from build123d import *

# Parameters (mm, degrees)
SKETCH_1_W      = 20
SKETCH_1_H      = 25
EXTRUDE_1_DEPTH = 4
FILLET_2_R      = 1
FILLET_3_R      = 1


with BuildPart() as part:
    # 草图1 → 凸台-拉伸1 (new body)
    with BuildSketch(Plane(origin=(0, 0, 0), x_dir=(1, 0, 0), z_dir=(0, 1, 0))):
        Rectangle(SKETCH_1_W, SKETCH_1_H)
    extrude(amount=EXTRUDE_1_DEPTH)

    # 圆角2
    fillet_2_edges = [part.edges().sort_by_distance(p)[0] for p in [
        (-10, 4, 0),
        (0, 0, 12.5),
        (-10, 0, 0),
        (0, 0, -12.5),
        (10, 0, 0),
        (-10, 2, 12.5),
        (-10, 2, -12.5),
    ]]
    fillet(fillet_2_edges, radius=FILLET_2_R)

    # 圆角3
    # the kernel refuses this fillet: 1 mm, written as the material it takes off along each edge
    with BuildSketch(Plane(origin=(-9, 3, 11.5), x_dir=(0, 0, 1), z_dir=(0, 1, 0))) as fillet_3_piece_1_section:
        Polygon((0, 0), (FILLET_3_R, 0), (FILLET_3_R, -FILLET_3_R), (0, -FILLET_3_R), align=None)
    fillet_3_piece_1 = extrude(amount=FILLET_3_R, mode=Mode.PRIVATE)
    fillet_3_piece_1 = fillet_3_piece_1 - Plane(origin=(-9, 3, 11.5), x_dir=(0.7071067811865475, 0, -0.7071067811865477), z_dir=(0, 1, 0)) * Sphere(FILLET_3_R, mode=Mode.PRIVATE)
    add(fillet_3_piece_1, mode=Mode.SUBTRACT)
    with BuildSketch(Plane(origin=(-9, 3, -11.5), x_dir=(0, 1, 0), z_dir=(0, 0, -1))) as fillet_3_piece_2_section:
        Polygon((0, 0), (FILLET_3_R, 0), (FILLET_3_R, -FILLET_3_R), (0, -FILLET_3_R), align=None)
    fillet_3_piece_2 = extrude(amount=FILLET_3_R, mode=Mode.PRIVATE)
    fillet_3_piece_2 = fillet_3_piece_2 - Plane(origin=(-9, 3, -11.5), x_dir=(0.7071067811865475, -0.7071067811865475, 0), z_dir=(0, 0, -1)) * Sphere(FILLET_3_R, mode=Mode.PRIVATE)
    add(fillet_3_piece_2, mode=Mode.SUBTRACT)
    with BuildSketch(Plane(origin=(9, 1, 11.5), x_dir=(0, 0, 1), z_dir=(1, 0, 0))) as fillet_3_piece_3_section:
        Polygon((0, 0), (FILLET_3_R, 0), (FILLET_3_R, FILLET_3_R), (0, FILLET_3_R), align=None)
    fillet_3_piece_3 = extrude(amount=FILLET_3_R, mode=Mode.PRIVATE)
    fillet_3_piece_3 = fillet_3_piece_3 - Plane(origin=(9, 1, 11.5), x_dir=(0, 0.7071067811865475, -0.7071067811865475), z_dir=(1, 0, 0)) * Sphere(FILLET_3_R, mode=Mode.PRIVATE)
    add(fillet_3_piece_3, mode=Mode.SUBTRACT)
    with BuildSketch(Plane(origin=(9, 1, -11.5), x_dir=(1, 0, 0), z_dir=(0, 0, -1))) as fillet_3_piece_4_section:
        Polygon((0, 0), (FILLET_3_R, 0), (FILLET_3_R, FILLET_3_R), (0, FILLET_3_R), align=None)
    fillet_3_piece_4 = extrude(amount=FILLET_3_R, mode=Mode.PRIVATE)
    fillet_3_piece_4 = fillet_3_piece_4 - Plane(origin=(9, 1, -11.5), x_dir=(-0.7071067811865475, 0.7071067811865475, 0), z_dir=(0, 0, -1)) * Sphere(FILLET_3_R, mode=Mode.PRIVATE)
    add(fillet_3_piece_4, mode=Mode.SUBTRACT)
    with BuildSketch(Plane(origin=(9, 3, 11.5), x_dir=(0, 1, 0), z_dir=(1, 0, 0))) as fillet_3_piece_5_section:
        Polygon((0, 0), (FILLET_3_R, 0), (FILLET_3_R, FILLET_3_R), (0, FILLET_3_R), align=None)
    fillet_3_piece_5 = extrude(amount=FILLET_3_R, mode=Mode.PRIVATE)
    fillet_3_piece_5 = fillet_3_piece_5 - Plane(origin=(9, 3, 11.5), x_dir=(0, -0.7071067811865475, -0.7071067811865475), z_dir=(1, 0, 0)) * Sphere(FILLET_3_R, mode=Mode.PRIVATE)
    add(fillet_3_piece_5, mode=Mode.SUBTRACT)
    with BuildSketch(Plane(origin=(9, 3, -11.5), x_dir=(1, 0, 0), z_dir=(0, 0, -1))) as fillet_3_piece_6_section:
        Polygon((0, 0), (FILLET_3_R, 0), (FILLET_3_R, -FILLET_3_R), (0, -FILLET_3_R), align=None)
    fillet_3_piece_6 = extrude(amount=FILLET_3_R, mode=Mode.PRIVATE)
    fillet_3_piece_6 = fillet_3_piece_6 - Plane(origin=(9, 3, -11.5), x_dir=(-0.7071067811865475, -0.7071067811865475, 0), z_dir=(0, 0, -1)) * Sphere(FILLET_3_R, mode=Mode.PRIVATE)
    add(fillet_3_piece_6, mode=Mode.SUBTRACT)
    with BuildSketch(Plane(origin=(9, 4, 12.5), x_dir=(0, 0, -1), z_dir=(-1, 0, 0))) as fillet_3_piece_7:
        with BuildLine():
            CenterArc((FILLET_3_R, FILLET_3_R), FILLET_3_R, 180, 90)
            Line((0, FILLET_3_R), (0, 0))
            Line((0, 0), (FILLET_3_R, 0))
        make_face()
    extrude(amount=18, mode=Mode.SUBTRACT)
    with BuildSketch(Plane(origin=(10, 4, -11.5), x_dir=(0, -1, 0), z_dir=(0, 0, 1))) as fillet_3_piece_8:
        with BuildLine():
            CenterArc((FILLET_3_R, -FILLET_3_R), FILLET_3_R, 90, 90)
            Line((0, -FILLET_3_R), (0, 0))
            Line((0, 0), (FILLET_3_R, 0))
        make_face()
    extrude(amount=23, mode=Mode.SUBTRACT)
    with BuildSketch(Plane(origin=(-9, 4, -12.5), x_dir=(0, -1, 0), z_dir=(1, 0, 0))) as fillet_3_piece_9:
        with BuildLine():
            CenterArc((FILLET_3_R, -FILLET_3_R), FILLET_3_R, 90, 90)
            Line((0, -FILLET_3_R), (0, 0))
            Line((0, 0), (FILLET_3_R, 0))
        make_face()
    extrude(amount=18, mode=Mode.SUBTRACT)
    with BuildSketch(Plane(origin=(10, 1, 12.5), x_dir=(0, 0, -1), z_dir=(0, 1, 0)), Plane(origin=(10, 1, -12.5), x_dir=(-1, 0, 0), z_dir=(0, 1, 0))) as fillet_3_piece_10:
        with BuildLine():
            CenterArc((FILLET_3_R, FILLET_3_R), FILLET_3_R, 180, 90)
            Line((0, FILLET_3_R), (0, 0))
            Line((0, 0), (FILLET_3_R, 0))
        make_face()
    extrude(amount=2, mode=Mode.SUBTRACT)


solid = part.part
Here's how the part is built. I have some questions about the finished solid (model axes, mm). Coordinates: 2 decimals unless noted, no trailing zeros. Write each loop counter-clockwise with the first axis right and the second up, starting at its lowest first coordinate (ties: lowest second). Pieces come first, ordered by that corner, then holes.
Item 1: I want a section at B-B on y = 3.5. Write out the boundary of the cut face in (x, z), and give its area (3 significant figures).
Item 2: If I drill on line 1 (X direction, y = 3.35, z = -5); line 2 (X direction, y = 3.15, z = -1.75); line 3 (Z direction, x = -5, y = 3.3), over which ranges is the centre line in solid material (lowest first)?
Item 3: I want a section at A-A on y = 0.4. Write out the boundary of the cut face in (x, z).
Findings below:
1. outline: (-9.87, -11.5) arc R0.87 ccw to (-9, -12.37) - (9, -12.37) arc R0.87 ccw to (9.87, -11.5) - (9.87, 11.5) arc R0.87 ccw to (9, 12.37) - (-9, 12.37) arc R0.87 ccw to (-9.87, 11.5) - close
1. area: 487 mm2
2. line 1: x = -9.94 to 9.94
2. line 2: x = -9.99 to 9.99
2. line 3: z = -12.45 to 12.45
3. outline: (-9.8, -11.5) arc R0.8 ccw to (-9, -12.3) - (9, -12.3) arc R0.8 ccw to (9.8, -11.5) - (9.8, 11.5) arc R0.8 ccw to (9, 12.3) - (-9, 12.3) arc R0.8 ccw to (-9.8, 11.5) - close
